from build123d import *

# Parameters (mm, degrees)
F0_W     = 40
F0_H     = 40
F1_DEPTH = 2
F2_W     = 35
F2_H     = 35
F3_DEPTH = 55
F4_W     = 31
F4_H     = 31
F5_DEPTH = 57.001
F6_R     = 1
F8_DEPTH = 55


with BuildPart() as f1:
    # F0 (on Top) → F1 (new body)
    with BuildSketch(Plane.XY):
        with Locations((-3.9790219205, -2.1009873599)):
            Rectangle(F0_W, F0_H)
    extrude(amount=F1_DEPTH)

    # F2 (on face) → F3 (join)
    with BuildSketch(Plane.XY.offset(2)):
        with Locations((-3.9790219205, -2.1009873599)):
            Rectangle(F2_W, F2_H)
    extrude(amount=F3_DEPTH)

    # F4 (on face) → F5 (cut, through all)
    with BuildSketch(Plane.XY.offset(57)):
        with Locations((-3.9790219205, -2.1009873599)):
            Rectangle(F4_W, F4_H)
    extrude(amount=-F5_DEPTH, mode=Mode.SUBTRACT)

    # F6
    f6_edges = [f1.edges().sort_by_distance(p)[0] for p in [
        (13.520978, -19.600987, 29.5),
        (13.520978, 15.399013, 29.5),
        (-21.479022, -19.600987, 29.5),
        (-21.479022, 15.399013, 29.5),
    ]]
    fillet(f6_edges, radius=F6_R)

    # F7 (on face) → F8 (cut, through all)
    with BuildSketch(Plane.XY.offset(57)):
        with BuildLine():
            Line((-6.0118580349, -19.6009873599), (-5.0118580349, -19.6009873599))
            ThreePointArc((-5.0118580349, -19.6009873599), (-5.5118580349, -19.1009873599), (-6.0118580349, -19.6009873599))
        make_face()
    extrude(amount=-F8_DEPTH, mode=Mode.SUBTRACT)


solid = f1.part
Input: part model. Units: mm. Frame: model coordinates. A direction names the side the tool comes from. Coordinates: 2 decimals unless noted, no trailing zeros. Order: outer loops, then holes, each group sorted by start corner. A loop starts at its lowest first (then second) coordinate and runs counter-clockwise, first axis right, second up.
1. Cut plane A-A, the plane x = 1. Return loops of the section in (y, z), plus the area to 3 significant figures.
Checked values:
outline: (-22.1, 0) - (-17.6, 0) - (-17.6, 57) - (-19.6, 57) - (-19.6, 2) - (-22.1, 2) - close; (13.4, 0) - (17.9, 0) - (17.9, 2) - (15.4, 2) - (15.4, 57) - (13.4, 57) - close
area: 238 mm2
2. Access query for faces 4 (the flat face through (13.521, -2, 29)), 5 (the flat face through (-19.479, -2, 29)), 6 (the flat face through (-4, 15.399, 29)), 7 (the flat face through (-22, -2, 2)), 8 (the flat face through (4, -19.601, 29)). Directions: +Z, -Z, +X, -X, +Y, -Y. A direction counts if a zero-diameter tool reaches every point of the face in a straight line with its end or side. Return the directions, or none.
Checked values:
face 4: +Z, +X, +Y, -Y
face 5: +Z, -Z
face 6: +Z, +X, -X, +Y
face 7: +Z
face 8: +Z, +X, -X, -Y
3. Cut plane C-C, the plane z = 38.5. Return loops of the section in (x, y), plus the area to 3 significant figures.
Checked values:
outline: (-21.48, -18.6) arc R1 ccw to (-20.48, -19.6) - (-6.01, -19.6) arc R0.5 cw to (-5.01, -19.6) - (12.52, -19.6) arc R1 ccw to (13.52, -18.6) - (13.52, 14.4) arc R1 ccw to (12.52, 15.4) - (-20.48, 15.4) arc R1 ccw to (-21.48, 14.4) - close; hole (-19.48, -17.6) - (11.52, -17.6) - (11.52, 13.4) - (-19.48, 13.4) - close
area: 263 mm2
4. Contact query for flat-ended pins moving along their axis: P1, Ø4, axis at x = -18, z = 33, coming from the -Y side; P2, Ø10, axis at y = -6.5, z = 21, coming from the -X side; P3, Ø15.5, axis at x = -11.5, z = 41, coming from the +Y side; P4, Ø2, axis at x = -2.5, y = 11, coming from the -Z side. Output: stop coordinate, or through.
Checked values:
P1: stops at y = -19.6
P2: stops at x = -21.48
P3: stops at y = 15.4
P4: passes through
5. Cut plane B-B, the plane y = -15. Return loops of the section in (x, z).
Checked values:
outline: (-23.98, 0) - (-19.48, 0) - (-19.48, 57) - (-21.48, 57) - (-21.48, 2) - (-23.98, 2) - close; (11.52, 0) - (16.02, 0) - (16.02, 2) - (13.52, 2) - (13.52, 57) - (11.52, 57) - close
6. Draft query along X for faces 1 (the flat face through (11.521, -2, 29)), 2 (the flat face through (-4, 17.899, 1)), 3 (the flat face through (-21.479, -2, 29)). Return one class per face: +X half, -X half, draft (parallel to the pull), parting line (faces both ways), or undercut.
Checked values:
face 1: undercut
face 2: draft
face 3: -X half
7. Ray query, line 1 along X through (y, z) = (-8.5, 33); line 2 along Y through (x, z) = (-9, 8); line 3 along Z through (x, y) = (-22, 15). Return the intervals inside material, ascending.
Checked values:
line 1: x = -21.48 to -19.48, 11.52 to 13.52
line 2: y = -19.6 to -17.6, 13.4 to 15.4
line 3: z = 0 to 2
